Read the model definition and answer for the solid it produces. Units are mm, in the model's axes. A direction names the side the tool comes from. Give positions to 0.01 mm unless a question says otherwise; leave off trailing zeros. Order: outer loops, then holes, each group sorted by start corner. A loop starts at its lowest first (then second) coordinate and runs counter-clockwise, first axis right, second up. Notation, with made-up numbers: (25, -3.5) - (65, -3.5) arc R11 ccw to (65, 9.5) - close; hole circle Ø9 at (42.25, 74). An arc over 180 degrees is marked (long way). Use a Markdown table: item, result. Add a question column.
1. A cutting plane is placed at B-B on y = -4.5. Determine the outline of the cut face in (x, z) (3 decimals).
2. A cutting plane is placed at A-A on x = 0. Determine the outline of the cut face in (y, z) (3 decimals).
3. Which of the six approach directions +Z, -Z, +X, -X, +Y, -Y give full straight-line access (tool end or side, diameter ignored) to faces 4 (the flat face through (39, 3, -12.7)), 5 (the flat face through (10.3, -3.26, -20.76)), 6 (the flat face through (-12.7, 3, 42))?
4. Consider L1, parallel to Z at x = 20.5, y = -3.75; L2, parallel to X at y = 3.75, z = -2; L3, parallel to Y at x = -11, z = 29. Determine where each line is inside the solid, lowest interval first.
5. Flat-ended cylindrical pins translate along their axes: P1, Ø7, axis at x = -39, y = 3, coming from the +Z side; P2, Ø1.9, axis at y = 3.5, z = 40, coming from the -X side; P3, Ø1.9, axis at x = -38.5, y = 1.5, coming from the -Z side. Find the tip coordinate at first contact, or state that the pin passes through.
6. A cutting plane is placed at C-C on y = 2. State how many separate pieces and enclosed holes the cut face has, and give its area (3 significant figures).
7. For a pull along X with two mould halves and no side action, classify faces 1 (the flat face through (-20.76, -3.26, -10.3)), 2 (the cylindrical face through (10.368, -0.072, 20.726)), 3 (the flat face through (0, -6.35, 24)) as released by +X, released by -X, zero draft, split by the parting line, or undercut.
8. A cutting plane is placed at D-D on z = 44. Determine the outline of the cut face in (x, y).
```python
from build123d import *

# Parameters (mm, degrees)
SKETCH1_R                    = 14.12875
STOCK_EXTRUDE_DEPTH          = 6.35
F_10_0_1935_DIAMETER_HOLE1_D = 4.9149
BOSS_EXTRUDE2_DEPTH          = 6.35
FILLET2_R                    = 2.54
FILLET3_R                    = 0.254
FILLET4_R                    = 2.54
F_10_0_1935_DIAMETER_HOLE2_D = 4.9149


with BuildPart() as part:
    # Sketch1 → Stock Extrude (new body)
    # profile 1 of 6: a face of its own
    with BuildSketch(Plane(origin=(0, 0, 0), x_dir=(1, 0, 0), z_dir=(0, 1, 0))):
        with BuildLine():
            Line((-45.234068682, -12.7), (-32.534068682, -12.7))
            ThreePointArc((-32.534068682, -12.7), (-34.925, 0), (-32.534068682, 12.7))
            Line((-32.534068682, 12.7), (-45.234068682, 12.7))
            Line((-45.234068682, 12.7), (-45.234068682, -12.7))
        make_face()
    # profile 2 of 6: a face of its own
    with BuildSketch(Plane(origin=(0, 0, 0), x_dir=(1, 0, 0), z_dir=(0, 1, 0))):
        with BuildLine():
            Line((-12.7, -32.534068682), (12.7, -32.534068682))
            ThreePointArc((12.7, -32.534068682), (24.695704333, -24.695704333), (32.534068682, -12.7))
            ThreePointArc((32.534068682, -12.7), (34.322062684, -6.461550754), (34.925, 0))
            ThreePointArc((34.925, 0), (34.322062684, 6.461550754), (32.534068682, 12.7))
            ThreePointArc((32.534068682, 12.7), (0, 34.925), (-32.534068682, 12.7))
            Line((-32.534068682, 12.7), (-32.534068682, -12.7))
            ThreePointArc((-32.534068682, -12.7), (-24.695704333, -24.695704333), (-12.7, -32.534068682))
        make_face()
        with Locations(Location((0, 0, 0), (0, 0, 270))):
            Circle(SKETCH1_R, mode=Mode.SUBTRACT)
    # profile 3 of 6: a face of its own
    with BuildSketch(Plane(origin=(0, 0, 0), x_dir=(1, 0, 0), z_dir=(0, 1, 0))):
        with BuildLine():
            ThreePointArc((34.925, 0), (34.322062684, -6.461550754), (32.534068682, -12.7))
            Line((32.534068682, -12.7), (45.234068682, -12.7))
            Line((45.234068682, -12.7), (45.234068682, 12.7))
            Line((45.234068682, 12.7), (32.534068682, 12.7))
            ThreePointArc((32.534068682, 12.7), (34.322062684, 6.461550754), (34.925, 0))
        make_face()
    # profile 4 of 6: a face of its own
    with BuildSketch(Plane(origin=(0, 0, 0), x_dir=(1, 0, 0), z_dir=(0, 1, 0))):
        with BuildLine():
            ThreePointArc((-32.534068682, 12.7), (-34.925, 0), (-32.534068682, -12.7))
            Line((-32.534068682, -12.7), (-32.534068682, 12.7))
        make_face()
    # profile 5 of 6: a face of its own
    with BuildSketch(Plane(origin=(0, 0, 0), x_dir=(1, 0, 0), z_dir=(0, 1, 0))):
        with BuildLine():
            Line((-12.7, -51.584068682), (12.7, -51.584068682))
            Line((12.7, -51.584068682), (12.7, -32.534068682))
            ThreePointArc((12.7, -32.534068682), (0, -34.925), (-12.7, -32.534068682))
            Line((-12.7, -32.534068682), (-12.7, -51.584068682))
        make_face()
    # profile 6 of 6: a face of its own
    with BuildSketch(Plane(origin=(0, 0, 0), x_dir=(1, 0, 0), z_dir=(0, 1, 0))):
        with BuildLine():
            ThreePointArc((-12.7, -32.534068682), (0, -34.925), (12.7, -32.534068682))
            Line((12.7, -32.534068682), (-12.7, -32.534068682))
        make_face()
    extrude(amount=STOCK_EXTRUDE_DEPTH)

    # #10 (0.1935) Diameter Hole1 (through all)
    with Locations(Plane(origin=(0, 6.35, 0), x_dir=(1, 0, 0), z_dir=(0, 1, 0))):
        with Locations((-17.960512242, 17.960512242), (17.960512242, 17.960512242), (-17.960512242, -17.960512242), (17.960512242, -17.960512242)):
            Hole(F_10_0_1935_DIAMETER_HOLE1_D / 2)

    # Sketch4 → Boss-Extrude2 (add)
    with BuildSketch(Plane.XZ):
        with BuildLine():
            ThreePointArc((-26.735172091, 13.264787909), (-29.845, 0), (-26.735172091, -13.264787909))
            Line((-26.735172091, -13.264787909), (-17.065003462, -8.466885899))
            ThreePointArc((-17.065003462, -8.466885899), (-19.05, 0), (-17.065003462, 8.466885899))
            Line((-17.065003462, 8.466885899), (-26.735172091, 13.264787909))
        make_face()
        with BuildLine():
            Line((26.735172091, 13.264787909), (17.065003462, 8.466885899))
            ThreePointArc((17.065003462, 8.466885899), (18.547113198, 4.348228607), (19.05, 0))
            ThreePointArc((19.05, 0), (18.547113198, -4.348228607), (17.065003462, -8.466885899))
            Line((17.065003462, -8.466885899), (26.735172091, -13.264787909))
            ThreePointArc((26.735172091, -13.264787909), (29.05714401, -6.812224818), (29.845, 0))
            ThreePointArc((29.845, 0), (29.05714401, 6.812224818), (26.735172091, 13.264787909))
        make_face()
        with BuildLine():
            Line((-8.466885899, -17.065003462), (-13.264787909, -26.735172091))
            ThreePointArc((-13.264787909, -26.735172091), (0, -29.845), (13.264787909, -26.735172091))
            Line((13.264787909, -26.735172091), (8.466885899, -17.065003462))
            ThreePointArc((8.466885899, -17.065003462), (0, -19.05), (-8.466885899, -17.065003462))
        make_face()
        with BuildLine():
            ThreePointArc((13.264787909, 26.735172091), (0, 29.845), (-13.264787909, 26.735172091))
            Line((-13.264787909, 26.735172091), (-8.466885899, 17.065003462))
            ThreePointArc((-8.466885899, 17.065003462), (0, 19.05), (8.466885899, 17.065003462))
            Line((8.466885899, 17.065003462), (13.264787909, 26.735172091))
        make_face()
    extrude(amount=BOSS_EXTRUDE2_DEPTH)

    # Fillet2
    fillet2_edges = [part.edges().sort_by_distance(p)[0] for p in [
        (-26.735172091, -3.175, 13.264787909),
        (-26.735172091, -3.175, -13.264787909),
        (13.264787909, -3.175, 26.735172091),
        (-13.264787909, -3.175, 26.735172091),
        (26.735172091, -3.175, -13.264787909),
        (26.735172091, -3.175, 13.264787909),
        (-13.264787909, -3.175, -26.735172091),
        (13.264787909, -3.175, -26.735172091),
    ]]
    fillet(fillet2_edges, radius=FILLET2_R)

    # Fillet3
    fillet3_edges = [part.edges().sort_by_distance(p)[0] for p in [
        (-20.709391169, 0, -10.275066892),
        (-29.845, 0, 0),
        (0, 0, 29.845),
        (29.845, 0, 0),
        (20.70939117, 0, -10.275066892),
        (0, 0, -29.845),
        (-10.275066892, 0, -20.709391169),
        (10.275066892, 0, -20.709391169),
        (-26.404539016, 0, -12.174727831),
        (-26.404539016, 0, 12.174727831),
        (-12.174727831, 0, 26.404539016),
        (12.174727831, 0, 26.404539016),
        (26.404539016, 0, 12.174727831),
        (26.404539016, 0, -12.174727831),
        (-12.174727831, 0, -26.404539016),
        (12.174727831, 0, -26.404539016),
        (-20.709391169, 0, 10.275066892),
        (10.275066892, 0, 20.70939117),
        (-10.275066892, 0, 20.70939117),
        (20.70939117, 0, 10.275066892),
    ]]
    fillet(fillet3_edges, radius=FILLET3_R)

    # Fillet4
    fillet4_edges = [part.edges().sort_by_distance(p)[0] for p in [
        (-45.234068682, 3.175, 12.7),
        (-45.234068682, 3.175, -12.7),
        (-32.534068682, 3.175, -12.7),
        (32.534068682, 3.175, -12.7),
        (45.234068682, 3.175, -12.7),
        (45.234068682, 3.175, 12.7),
        (32.534068682, 3.175, 12.7),
        (12.7, 3.175, 32.534068682),
        (12.7, 3.175, 51.584068682),
        (-12.7, 3.175, 51.584068682),
        (-12.7, 3.175, 32.534068682),
        (-32.534068682, 3.175, 12.7),
    ]]
    fillet(fillet4_edges, radius=FILLET4_R)

    # #10 (0.1935) Diameter Hole2 (through all)
    with Locations(Plane(origin=(0, 6.35, 0), x_dir=(1, 0, 0), z_dir=(0, 1, 0))):
        with Locations((-36.979068682, 0)):
            Hole(F_10_0_1935_DIAMETER_HOLE2_D / 2)


solid = part.part
```
Output values:
| question | item | result |
|---|---|---|
| 1 | outline | (-27.853, -10.72) arc R2.54 ccw to (-24.354, -12.083) - (-17.065, -8.467) arc R19.05 cw to (-17.065, 8.467) - (-24.354, 12.083) arc R2.54 ccw to (-27.853, 10.72) arc R29.845 ccw to start; (-12.083, -24.354) arc R2.54 ccw to (-10.72, -27.853) arc R29.845 ccw to (10.72, -27.853) arc R2.54 ccw to (12.083, -24.354) - (8.467, -17.065) arc R19.05 cw to (-8.467, -17.065) - close; (-12.083, 24.354) - (-8.467, 17.065) arc R19.05 cw to (8.467, 17.065) - (12.083, 24.354) arc R2.54 ccw to (10.72, 27.853) arc R29.845 ccw to (-10.72, 27.853) arc R2.54 ccw to start; (17.065, -8.467) - (24.354, -12.083) arc R2.54 ccw to (27.853, -10.72) arc R29.845 ccw to (27.853, 10.72) arc R2.54 ccw to (24.354, 12.083) - (17.065, 8.467) arc R19.05 cw to start |
| 2 | outline | (-6.35, -29.845) - (-0.254, -29.845) arc R0.254 cw to (0, -30.099) - (0, -34.925) - (6.35, -34.925) - (6.35, -14.129) - (0, -14.129) - (0, -19.05) - (-6.35, -19.05) - close; (-6.35, 19.05) - (0, 19.05) - (0, 14.129) - (6.35, 14.129) - (6.35, 51.584) - (0, 51.584) - (0, 30.099) arc R0.254 cw to (-0.254, 29.845) - (-6.35, 29.845) - close |
| 3 | face 4 | -Z, +X, +Y, -Y |
| 3 | face 5 | +X, -Y |
| 3 | face 6 | +Z, -X, +Y, -Y |
| 4 | L1 | -10.17 to 10.17 |
| 4 | L2 | -45.23 to -38.41, -35.55 to -13.99, 13.99 to 45.23 |
| 4 | L3 | 0 to 6.35 |
| 5 | P1 | z = 12.7 |
| 5 | P2 | x = -12.7 |
| 5 | P3 | z = -12.7 |
| 6 | separate pieces | 1 |
| 6 | enclosed holes | 6 |
| 6 | area | 4,110 mm² |
| 7 | face 1 | undercut |
| 7 | face 2 | released by +X |
| 7 | face 3 | zero draft |
| 8 | outline | (-12.7, 0) - (12.7, 0) - (12.7, 6.35) - (-12.7, 6.35) - close |
